For this review, take the finished solid that the model builds, in its own axes (mm). Coordinates: 2 decimals unless noted, no trailing zeros. Loops run counter-clockwise (first coordinate to the right, second up) from the corner with the lowest first, then second, coordinate; pieces in that order, holes last. Notation, with made-up numbers: (67.5, 29) -> (126.5, 29) arc R15 ccw to (126.5, 41) -> close; hole circle Ø3 at (-34, 78.5). An arc over 180 degrees is marked (long way). Answer in a Markdown table with one row per item.
from build123d import *

# Parameters (mm, degrees)
ESQUISSE1_R        = 4
ESQUISSE1_R_2      = 2
BOSS_EXTRU_1_DEPTH = 10
CONG_1_R           = 10


with BuildPart() as part:
    # Esquisse1 → Boss.-Extru.1 (new body)
    with BuildSketch(Plane.XY):
        Polygon((0, 20), (0, 0), (60, 0), (154, 0), (174, 0), (174, 20), (154, 20), (60, 20), align=None)
        with Locations((10, 10)):
            Circle(ESQUISSE1_R, mode=Mode.SUBTRACT)
        with Locations((54, 10)):
            Circle(ESQUISSE1_R, mode=Mode.SUBTRACT)
        with Locations((154, 10)):
            Circle(ESQUISSE1_R_2, mode=Mode.SUBTRACT)
        with Locations((164, 10)):
            Circle(ESQUISSE1_R_2, mode=Mode.SUBTRACT)
        with Locations((74, 10)):
            Circle(ESQUISSE1_R_2, mode=Mode.SUBTRACT)
        with Locations((94, 10)):
            Circle(ESQUISSE1_R_2, mode=Mode.SUBTRACT)
        with Locations((114, 10)):
            Circle(ESQUISSE1_R_2, mode=Mode.SUBTRACT)
        with Locations((134, 10)):
            Circle(ESQUISSE1_R_2, mode=Mode.SUBTRACT)
    extrude(amount=BOSS_EXTRU_1_DEPTH)

    # Congé1
    cong_1_edges = [part.edges().sort_by_distance(p)[0] for p in [
        (0, 0, 5),
        (0, 20, 5),
        (174, 0, 5),
        (174, 20, 5),
    ]]
    fillet(cong_1_edges, radius=CONG_1_R - 0.0001)  # a hair under: the kernel refuses the full size


solid = part.part
Item 1: Take a section at B-B, the plane z = 4. Count the separate pieces of the cut face and the enclosed holes in it, and give its area (3 significant figures).
Worked answers:
| item | result |
|---|---|
| separate pieces | 1 |
| enclosed holes | 8 |
| area | 3,220 mm² |
Item 2: Take a section at C-C, the plane y = 3. State the section outline as (x, z) points.
Worked answers:
| item | result |
|---|---|
| outline | (2.86, 0) -> (171.14, 0) -> (171.14, 10) -> (2.86, 10) -> close |
Item 3: Insertion check: pin 1 (4 mm diameter, centred on y = 13.5, z = 2.5, fed in from +X); pin 2 (1 mm diameter, centred on y = 11, z = 6, fed in from -X). Each pin has a flat end and moves straight along its axis. Give the tip position at first contact, or say it passes through.
Worked answers:
| item | result |
|---|---|
| pin 1 | x = 173.89 |
| pin 2 | x = 0.01 |
Item 4: Take a section at A-A, the plane x = 114. State the section outline as (y, z) points, and give its area (3 significant figures).
Worked answers:
| item | result |
|---|---|
| outline | (0, 0) -> (8, 0) -> (8, 10) -> (0, 10) -> close; (12, 0) -> (20, 0) -> (20, 10) -> (12, 10) -> close |
| area | 160 mm² |
Item 5: The part is to be moulded in two halves that separate along X. For faces 1 (the cylindrical face through (75.908, 10.601, 4.93)), 2 (the cylindrical face through (170.99, 2.85, 5.07)), 3 (the flat face through (88, 20, 5)), say which applies: +X half, -X half, draft (parallel to the pull), parting line (faces both ways), or undercut.
Worked answers:
| item | result |
|---|---|
| face 1 | undercut |
| face 2 | +X half |
| face 3 | draft |
Item 6: For L1, parallel to Y at x = 74, z = 3; L2, parallel to Y at x = 10, z = 5; L3, parallel to X at y = 13.5, z = 1, list the stretches that pass through material, from the lowest coordinate up.
Worked answers:
| item | result |
|---|---|
| L1 | 0 to 8, 12 to 20 |
| L2 | 0 to 6, 14 to 20 |
| L3 | 0.63 to 8.06, 11.94 to 52.06, 55.94 to 173.37 |
